Autodesk Inventor part; units mm, degrees
ref_plane "YZ Plane" through (0, 0, 0) normal (1, 0, 0) x (0, 1, 0)
ref_plane "XZ Plane" through (0, 0, 0) normal (0, 1, 0) x (-1, 0, 0)
ref_plane "XY Plane" through (0, 0, 0) normal (0, 0, 1) x (1, 0, 0)
sketch "Sketch2" plane through (0, 0, 0) normal (0, 1, 0) x (-1, 0, 0)
  line L0 (-749.3, 508) -> (-749.3, -508)
  line L1 (-749.3, -508) -> (749.3, -508)
  line L2 (749.3, -508) -> (749.3, 508)
  line L3 (749.3, 508) -> (-749.3, 508)
  line L4 (-749.3, 508) -> (749.3, -508) construction
  line L5 (-749.3, -508) -> (749.3, 508) construction
  line L6 (-752.475, 511.175) -> (-752.475, -511.175)
  line L7 (-752.475, -511.175) -> (752.475, -511.175)
  line L8 (752.475, -511.175) -> (752.475, 511.175)
  line L9 (752.475, 511.175) -> (-752.475, 511.175)
  line L10 (-752.475, 511.175) -> (752.475, -511.175) construction
  line L11 (-752.475, -511.175) -> (752.475, 511.175) construction
  point P0 (0, 0)
  dimension "d4" = 1016
  dimension "d5" = 1498.6
  dimension "d6" = 3.175
  dimension "d7" = 3.175
extrude "Extrusion1" add sketch "Sketch2" along normal blind 1371.6
equation "\"d4\" = maxMatchWidth"
equation "\"d5\" = maxMatchLength"
equation "\"d6\" = modelThickness"
equation "\"d7\" = modelThickness"
equation "\"d8\" = maxMatchHeight"
equation "\"robotLength\" = 736.6"
equation "\"robotWidth\" = 254"
equation "\"robotPerimeter\" = 2 * robotLength + 2 * robotWidth"
equation "\"maxMatchLength\" = robotLength + 2 * matchExtension"
equation "\"matchExtension\" = 381"
equation "\"maxMatchWidth\" = robotWidth + 2 * matchExtension"
equation "\"modelThickness\" = 3.175"
equation "\"maxMatchHeight\" = 1371.6"
properties part number "RhinoV19MaxVolume" material "Polycarbonate, Smoke"
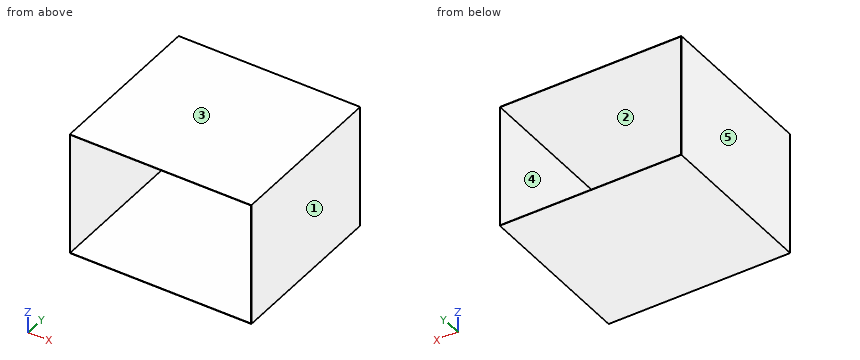
The model under review builds one solid part; all positions refer to its coordinate system, in mm. Face numbers are marked on the shaded views. A direction names the side the tool comes from. Coordinates: 2 decimals unless noted, no trailing zeros. Write each loop counter-clockwise with the first axis right and the second up, starting at its lowest first coordinate (ties: lowest second). Pieces come first, ordered by that corner, then holes. Notation, with made-up numbers: (55, 44.25) - (73, 44.25) arc R18 ccw to (73, 51.25) - close; hole circle Ø9 at (82.25, 36). An arc over 180 degrees is marked (long way). Write item = value, one per line.
(1) Machinability: for the marked faces 4 and 5, which of the approach directions +Z, -Z, +X, -X, +Y, -Y give a long, thin tool a straight path to every point of the face, cutting with its end or side? Answer none if there is none.
Result sheet:
face_4 = +Y, -Y
face_5 = +Z, -Z, -X, +Y, -Y
(2) Mouldability with a two-part tool opening along X and no side actions: class the marked faces 1, 2 and 3 as pulls with the +X half, pulls with the -X half, needs draft (parallel to the pull), parting line crosses it, or undercut.
Result sheet:
face_1 = pulls with the +X half
face_2 = undercut
face_3 = needs draft
(3) Consider section C-C, the plane x = 513. Give the boundary of the cut face in (y, z) (3 decimals).
Result sheet:
outline = (0, -511.175) - (1371.6, -511.175) - (1371.6, -508) - (0, -508) - close; (0, 508) - (1371.6, 508) - (1371.6, 511.175) - (0, 511.175) - close
(4) For line 1 (Z direction, x = 627.5, y = 763) (3 decimals); line 2 (X direction, y = 1255, z = 102.5) (3 decimals), list the stretches that pass through material, from the lowest coordinate up. Write a range as [from, to].
Result sheet:
line_1 = [-511.175, -508], [508, 511.175]
line_2 = [-752.475, -749.3], [749.3, 752.475]
(5) Consider section A-A, the plane z = 248.5. Give the boundary of the cut face in (x, y) (3 decimals), then the cut area to 3 significant figures.
Result sheet:
outline = (-752.475, 0) - (-749.3, 0) - (-749.3, 1371.6) - (-752.475, 1371.6) - close; (749.3, 0) - (752.475, 0) - (752.475, 1371.6) - (749.3, 1371.6) - close
area = 8,710 mm^2
(6) Consider section B-B, the plane y = 113.5. Give the boundary of the cut face in (x, z) (3 decimals), then the cut area to 3 significant figures.
Result sheet:
outline = (-752.475, -511.175) - (752.475, -511.175) - (752.475, 511.175) - (-752.475, 511.175) - close; hole (-749.3, -508) - (749.3, -508) - (749.3, 508) - (-749.3, 508) - close
area = 16,000 mm^2
